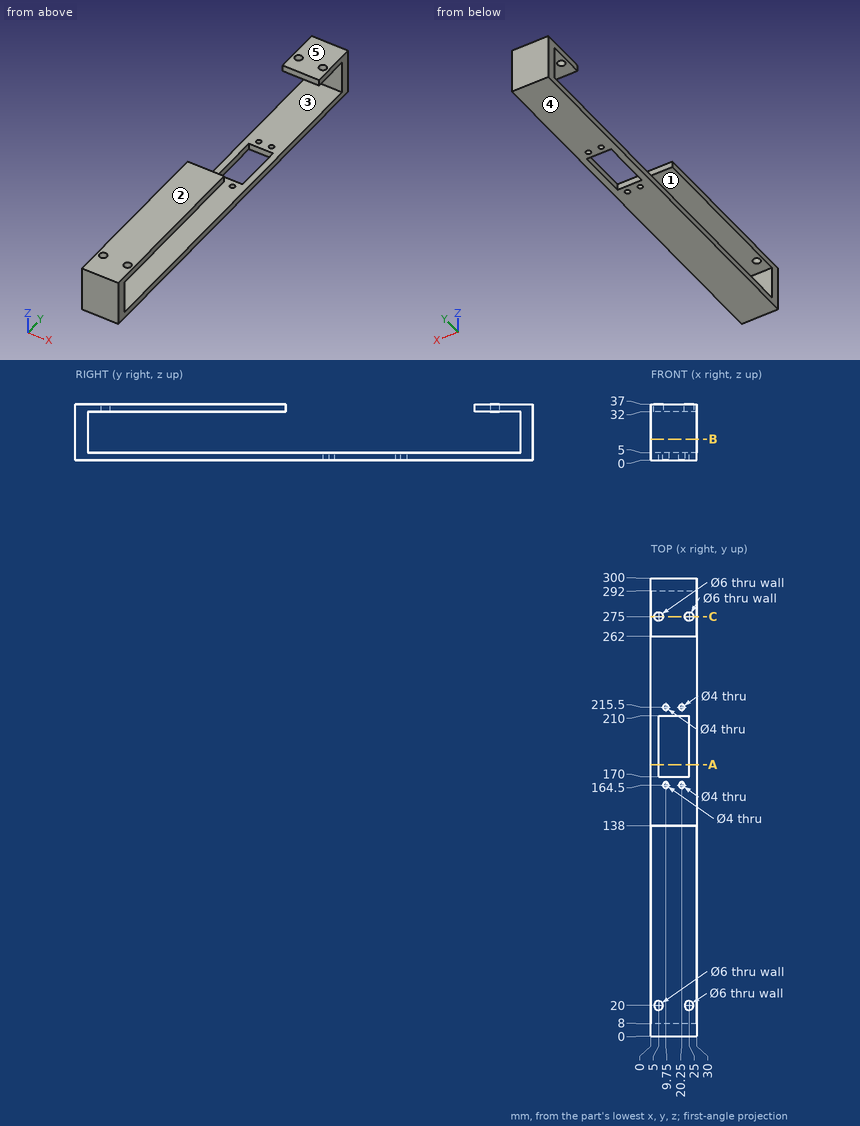
The drawing under review shows one solid part. Ordinate dimensions are in mm from its lowest x, y, z. A direction names the side the tool comes from. Coordinates: 2 decimals unless noted, no trailing zeros. Order: outer loops, then holes, each group sorted by start corner. A loop starts at its lowest first (then second) coordinate and runs counter-clockwise, first axis right, second up. Notation, with made-up numbers: (-30, 29) -> (-19, 29) arc R18 ccw to (-19, 41) -> close; hole circle Ø8 at (-10.5, -9). An arc over 180 degrees is marked (long way). Answer in a Markdown table with one row per item. Add a question column.
Item 1: Machinability: for the marked faces 1 and 2, which of the approach directions +Z, -Z, +X, -X, +Y, -Y give a long, thin tool a straight path to every point of the face, cutting with its end or side? Answer none if there is none.
Item 2: Clearance check with flat-ended pins moving along their axes: pin 1 (6 mm diameter, centred on y = 50, z = 9, fed in from +X); pin 2 (3.5 mm diameter, centred on x = 25, y = 20, fed in from +Z). State where each tip first meets the part, or that it passes through.
Item 3: We need section B-B on z = 14. Write out the cut boundary in (x, y), plus the area to 3 significant figures.
Item 4: Mouldability with a two-part tool opening along Z and no side actions: class the marked faces 3, 4 and 5 as +Z half, -Z half, draft (parallel to the pull), parting line (faces both ways), or undercut.
Item 5: We need section A-A on y = 178. Write out the cut boundary in (x, z), plus the area to 3 significant figures.
Item 6: We need section C-C on y = 275. Write out the cut boundary in (x, z), plus the area to 3 significant figures.
Item 7: To check wall thickness, follow probe 1 along Y at (x, z) = (9.75, 3.3); probe 2 along X at (y, z) = (164.5, 2.8); probe 3 along X at (y, z) = (275, 35). State the ranges of each line that lie inside material, in increasing order.
Final values:
| question | item | result |
|---|---|---|
| 1 | face 1 | +X, -X |
| 1 | face 2 | +Z, +X, -X, +Y, -Y |
| 2 | pin 1 | passes through |
| 2 | pin 2 | stops at z = 5 |
| 3 | outline | (0, 0) -> (30, 0) -> (30, 8) -> (0, 8) -> close; (0, 292) -> (30, 292) -> (30, 300) -> (0, 300) -> close |
| 3 | area | 480 mm2 |
| 4 | face 3 | undercut |
| 4 | face 4 | -Z half |
| 4 | face 5 | +Z half |
| 5 | outline | (0, 0) -> (5, 0) -> (5, 5) -> (0, 5) -> close; (25, 0) -> (30, 0) -> (30, 5) -> (25, 5) -> close |
| 5 | area | 50.0 mm2 |
| 6 | outline | (0, 0) -> (30, 0) -> (30, 5) -> (0, 5) -> close; (0, 32) -> (2, 32) -> (2, 37) -> (0, 37) -> close; (8, 32) -> (22, 32) -> (22, 37) -> (8, 37) -> close; (28, 32) -> (30, 32) -> (30, 37) -> (28, 37) -> close |
| 6 | area | 240 mm2 |
| 7 | probe 1 | y = 0 to 162.5, 166.5 to 170, 210 to 213.5, 217.5 to 300 |
| 7 | probe 2 | x = 0 to 7.75, 11.75 to 18.25, 22.25 to 30 |
| 7 | probe 3 | x = 0 to 2, 8 to 22, 28 to 30 |
